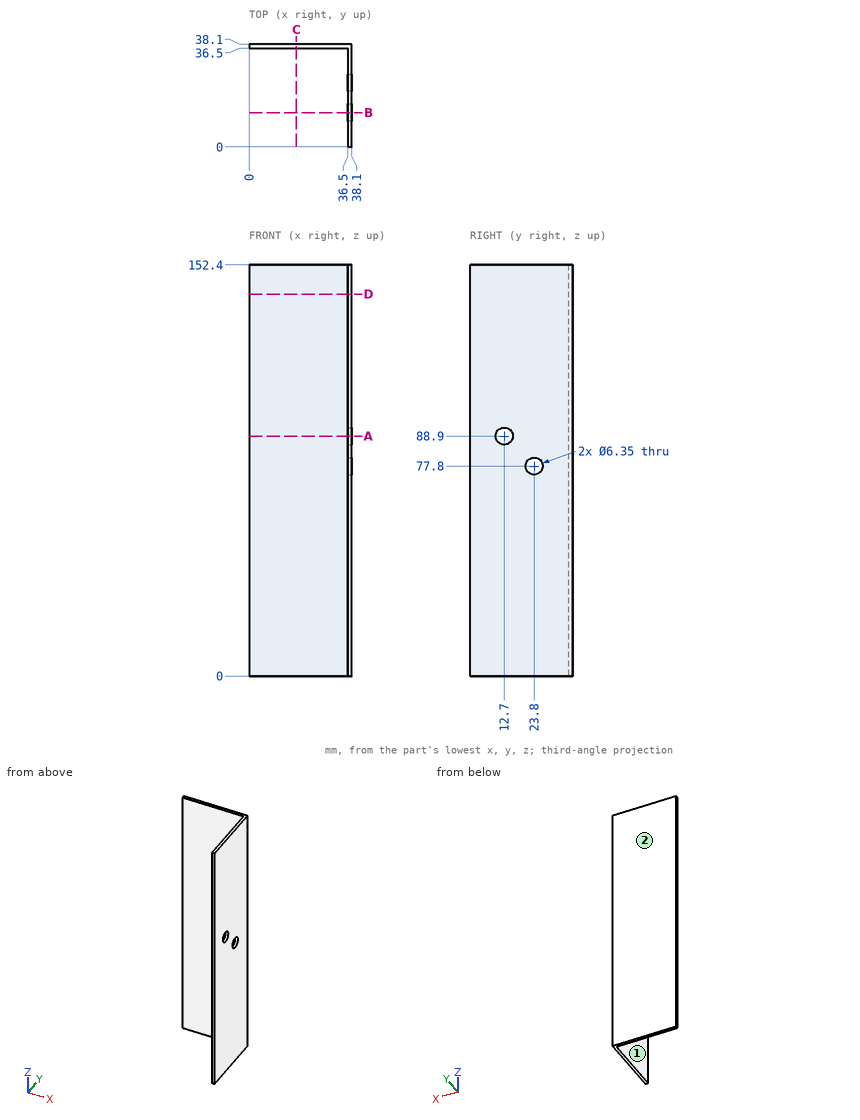
Could you check a few things on this drawing? It's one solid part, dimensions in mm from its lowest x, y, z. A direction names the side the tool comes from. Give positions to 0.01 mm unless a question says otherwise; leave off trailing zeros. Order: outer loops, then holes, each group sorted by start corner. A loop starts at its lowest first (then second) coordinate and runs counter-clockwise, first axis right, second up. Notation, with made-up numbers: (20, 88) - (71, 88) arc R7 ccw to (71, 94) - close; hole circle Ø3 at (8.5, 77). An arc over 180 degrees is marked (long way). Answer as a JSON object with one key per item and string values. Group by question number.
Item 1: For P1, Ø11, axis at y = 23, z = 104.5, coming from the -X side; P2, Ø18, axis at x = 24, z = 56.5, coming from the -Y side, each with a flat end and sliding along its axis, tell me the tip position at first contact or that it passes through.
Item 2: If we section it at B-B on y = 12.7: Please give me the cut outline in (x, z) (1 decimal).
Item 3: If we section it at C-C on x = 17.5: Please give me the cut outline in (y, z), and give its area (3 significant figures).
Item 4: Please list where these lines run through material, in increasing order: probe 1 along Y at (x, z) = (37.35, 88.9) (3 decimals); probe 2 along Y at (x, z) = (29.5, 46).
Item 5: Which directions (+Z, -Z, +X, -X, +Y, -Y) give clear straight access to the entire face, cutting with the end or side of a thin tool? Please do the marked faces 1 and 2.
Item 6: If we section it at A-A on z = 88.9: Please give me the cut outline in (x, y) (1 decimal), and give its area (3 significant figures).
Item 7: If we section it at D-D on z = 141.5: Please give me the cut outline in (x, y).
Result set:
{
 "1": {"P1": "x = 36.5", "P2": "y = 36.5"},
 "2": {"outline": "(36.5, 0) - (38.1, 0) - (38.1, 85.7) - (36.5, 85.7) - close; (36.5, 92.1) - (38.1, 92.1) - (38.1, 152.4) - (36.5, 152.4) - close"},
 "3": {"outline": "(36.5, 0) - (38.1, 0) - (38.1, 152.4) - (36.5, 152.4) - close", "area": "244 mm²"},
 "4": {"probe 1": "0 to 9.525, 15.875 to 38.1", "probe 2": "36.5 to 38.1"},
 "5": {"face 1": "+Z, -Z, -X, -Y", "face 2": "+Z, -Z, +X, -X, +Y"},
 "6": {"outline": "(0, 36.5) - (36.5, 36.5) - (36.5, 15.9) - (38.1, 15.9) - (38.1, 38.1) - (0, 38.1) - close; (36.5, 0) - (38.1, 0) - (38.1, 9.5) - (36.5, 9.5) - close", "area": "109 mm²"},
 "7": {"outline": "(0, 36.5) - (36.5, 36.5) - (36.5, 0) - (38.1, 0) - (38.1, 38.1) - (0, 38.1) - close"}
}
